```python
from build123d import *

# Parameters (mm, degrees)
F2_DEPTH = 63.5
F4_R     = 6.35
F5_DEPTH = 50.8


with BuildPart() as f2:
    # F1 (on Front) → F2 (new body, symmetric)
    with BuildSketch(Plane.XZ):
        Polygon((-63.5, 40.386), (-63.5, 0), (63.5, 0), (63.5, 40.386), (0, 40.386), align=None)
    extrude(amount=F2_DEPTH, both=True)

    # F0 (on Front) → F3 (revolve, cut)
    with BuildSketch(Plane.XZ):
        Polygon((0, 2.286), (0, 0), (38.1, 0), (91.416501, 0), (91.416501, 7.332348), (50.8, 7.332348), (46.840532, 7.332348), (38.1, 2.286), align=None)
    revolve(axis=Axis((0, 0, 1.143), (0, 0, -1)), mode=Mode.SUBTRACT)

    # F4 (on Top) → F5 (cut, symmetric)
    with BuildSketch(Plane.XY):
        with Locations((-50.8, 50.8)):
            Circle(F4_R)
        with Locations((50.8, -50.8)):
            Circle(F4_R)
    extrude(amount=F5_DEPTH, both=True, mode=Mode.SUBTRACT)


solid = f2.part
```
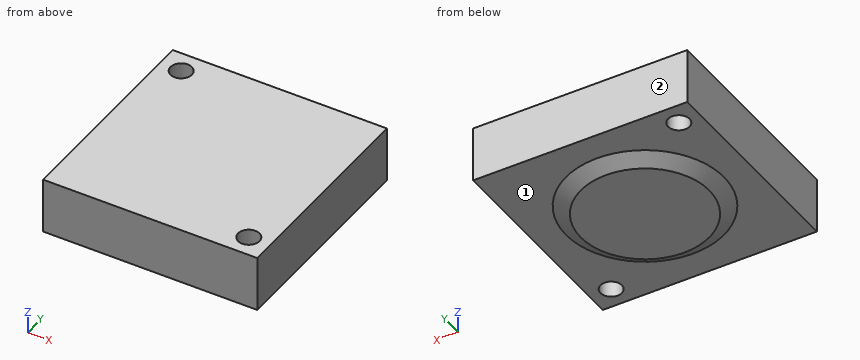
The model under review builds one solid part; all positions refer to its coordinate system, in mm. Face numbers are marked on the shaded views. A direction names the side the tool comes from. Give positions to 0.01 mm unless a question says otherwise; leave off trailing zeros. Write each loop counter-clockwise with the first axis right and the second up, starting at its lowest first coordinate (ties: lowest second). Pieces come first, ordered by that corner, then holes. Notation, with made-up numbers: M 36,-2 L 47,-2 A22 cw 47,31 Z; hole C -26,9 d10. An arc over 180 degrees is marked long. Answer in a Markdown table with one row per item.
Item 1: Add section C-C on z = 16. Give the boundary of the cut face in (x, y), plus the area to 3 significant figures.
Check sheet entries:
| item | result |
|---|---|
| outline | M -63.5,-63.5 L 63.5,-63.5 L 63.5,63.5 L -63.5,63.5 Z; hole C -50.8,50.8 d12.7; hole C 50.8,-50.8 d12.7 |
| area | 15,900 mm2 |
Item 2: For P1, Ø12, axis at x = 9.5, y = -43.5, coming from the -Z side; P2, Ø10, axis at x = 45, y = 41, coming from the -Z side; P3, Ø2, axis at x = 34, y = 29.5, coming from the -Z side, all flat-tipped, find the tip position at first contact; note any pin that passes through.
Check sheet entries:
| item | result |
|---|---|
| P1 | z = 2.53 |
| P2 | z = 7.33 |
| P3 | z = 5.7 |
Item 3: For line 1 along Y through (x, z) = (-50.8, 15.5); line 2 along Y through (x, z) = (50.8, 21); line 3 along Z through (x, y) = (-30.5, -39.5), list the stretches that pass through material, from the lowest coordinate up.
Check sheet entries:
| item | result |
|---|---|
| line 1 | -63.5 to 44.45, 57.15 to 63.5 |
| line 2 | -63.5 to -57.15, -44.45 to 63.5 |
| line 3 | 7.33 to 40.39 |
Item 4: Add section A-A on x = 50.8. Give the boundary of the cut face in (y, z).
Check sheet entries:
| item | result |
|---|---|
| outline | M -63.5,7.33 L -57.15,7.33 L -57.15,40.39 L -63.5,40.39 Z; M -44.45,7.33 L 63.5,7.33 L 63.5,40.39 L -44.45,40.39 Z |
Item 5: Add section D-D on y = 0. Give the boundary of the cut face in (x, z), plus the area to 3 significant figures.
Check sheet entries:
| item | result |
|---|---|
| outline | M -63.5,7.33 L -46.84,7.33 L -38.1,2.29 L 38.1,2.29 L 46.84,7.33 L 63.5,7.33 L 63.5,40.39 L -63.5,40.39 Z |
| area | 4,630 mm2 |
Item 6: Tool access review of the marked faces 1 and 2: name each direction out of +Z, -Z, +X, -X, +Y, -Y from which nothing blocks a thin tool from reaching the whole face with its end or side.
Check sheet entries:
| item | result |
|---|---|
| face 1 | -Z |
| face 2 | +Z, -Z, +X, -X, +Y |
